Geometry: final body of the model. Coordinates: model frame, mm. Face numbers are marked on the shaded views. A direction names the side the tool comes from. Round coordinates to 2 decimals unless told otherwise and drop trailing zeros. Loops run counter-clockwise (first coordinate to the right, second up) from the corner with the lowest first, then second, coordinate; pieces in that order, holes last. Notation, with made-up numbers: (80.5, -33.5) - (139.5, -33.5) arc R26 cw to (139.5, 0.5) - close; hole circle Ø9 at (45, 87). An arc over 180 degrees is marked (long way). Answer as CSV lines item,"result".
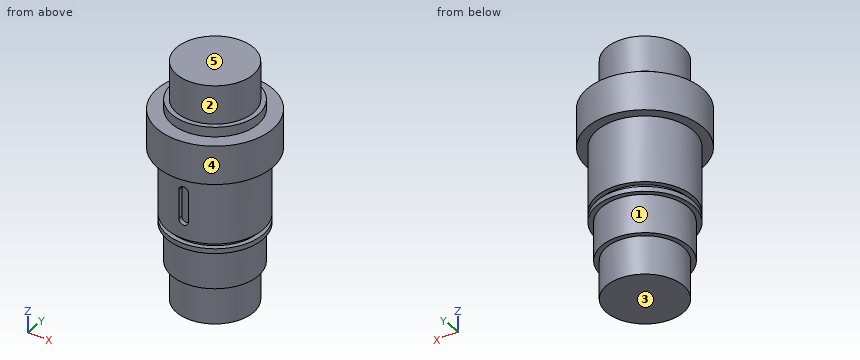
from build123d import *

# Parameters (mm, degrees)
SKETCH2_R           = 25.4
BOSS_EXTRUDE1_DEPTH = 25.4
SKETCH3_R           = 28.575
BOSS_EXTRUDE2_DEPTH = 25.4
SKETCH4_R           = 31.75
BOSS_EXTRUDE3_DEPTH = 3.175
SKETCH5_R           = 28.575
BOSS_EXTRUDE4_DEPTH = 3.175
SKETCH6_R           = 31.75
BOSS_EXTRUDE5_DEPTH = 43.5356
SKETCH7_R           = 38.1
BOSS_EXTRUDE6_DEPTH = 25.4
SKETCH8_R           = 28.575
BOSS_EXTRUDE7_DEPTH = 6.35
SKETCH9_R           = 25.4
BOSS_EXTRUDE8_DEPTH = 25.4
CUT_EXTRUDE1_DEPTH  = 3.175


with BuildPart() as part:
    # Sketch2 → Boss-Extrude1 (new body)
    with BuildSketch(Plane.XY):
        Circle(SKETCH2_R)
    extrude(amount=BOSS_EXTRUDE1_DEPTH)

    # Sketch3 → Boss-Extrude2 (add)
    with BuildSketch(Plane.XY.offset(25.4)):
        Circle(SKETCH3_R)
    extrude(amount=BOSS_EXTRUDE2_DEPTH)

    # Sketch4 → Boss-Extrude3 (add)
    with BuildSketch(Plane.XY.offset(50.8)):
        Circle(SKETCH4_R)
    extrude(amount=BOSS_EXTRUDE3_DEPTH)

    # Sketch5 → Boss-Extrude4 (add)
    with BuildSketch(Plane.XY.offset(53.975)):
        Circle(SKETCH5_R)
    extrude(amount=BOSS_EXTRUDE4_DEPTH)

    # Sketch6 → Boss-Extrude5 (add)
    with BuildSketch(Plane.XY.offset(57.15)):
        Circle(SKETCH6_R)
    extrude(amount=BOSS_EXTRUDE5_DEPTH)

    # Sketch7 → Boss-Extrude6 (add)
    with BuildSketch(Plane.XY.offset(100.6856)):
        Circle(SKETCH7_R)
    extrude(amount=BOSS_EXTRUDE6_DEPTH)

    # Sketch8 → Boss-Extrude7 (add)
    with BuildSketch(Plane.XY.offset(126.0856)):
        Circle(SKETCH8_R)
    extrude(amount=BOSS_EXTRUDE7_DEPTH)

    # Sketch9 → Boss-Extrude8 (add)
    with BuildSketch(Plane.XY.offset(132.4356)):
        Circle(SKETCH9_R)
    extrude(amount=BOSS_EXTRUDE8_DEPTH)

    # Sketch10 → Cut-Extrude1 (cut)
    with BuildSketch(Plane(origin=(0, -31.75, 0), x_dir=(-1, 0, 0), z_dir=(0, -1, 0))):
        with BuildLine():
            Line((3.175, -69.3928), (3.175, -88.4428))
            ThreePointArc((3.175, -88.4428), (0, -91.6178), (-3.175, -88.4428))
            Line((-3.175, -88.4428), (-3.175, -69.3928))
            ThreePointArc((-3.175, -69.3928), (0, -66.2178), (3.175, -69.3928))
        make_face()
    extrude(amount=-CUT_EXTRUDE1_DEPTH, mode=Mode.SUBTRACT)


solid = part.part
(1) Pin query (flat end, axial travel): P1, Ø10, axis at y = -29, z = 133.5, coming from the +X side; P2, Ø2, axis at x = -9.5, z = 21, coming from the -Y side; P3, Ø1.9, axis at x = 1, z = 81, coming from the -Y side (3 decimals). Return the tip coordinate at first contact, or that it passes through.
Findings below:
P1,"x = 15.33"
P2,"y = -23.94"
P3,"y = -28.575"
(2) Material intervals for line 1 along Z through (x, y) = (-33, 7); line 2 along Z through (x, y) = (-25.5, -6.5); line 3 along Z through (x, y) = (-31, -3.5) (3 decimals), sorted ascending.
Findings below:
line 1,"100.69 to 126.09"
line 2,"25.4 to 132.44"
line 3,"50.8 to 53.975, 57.15 to 126.086"
(3) Draft query along Y for the marked faces 4 and 5. Return one class per face: pulls with the +Y half, pulls with the -Y half, needs draft (parallel to the pull), parting line crosses it, or undercut.
Findings below:
face 4,"parting line crosses it"
face 5,"needs draft"
(4) Access query for the marked faces 1, 2 and 3. Directions: +Z, -Z, +X, -X, +Y, -Y. A direction counts if a zero-diameter tool reaches every point of the face in a straight line with its end or side. Return the directions, or none.
Findings below:
face 1,"-Z"
face 2,"+Z"
face 3,"-Z, +X, -X, +Y, -Y"
(5) Section B-B (z = 108.5). Output: boundary loops of the cut face in (x, y).
Findings below:
outline,"circle Ø76.2 at (0, 0)"
